```python
from build123d import *

# Parameters (mm, degrees)
F0_W     = 220
F0_H     = 163.86598641
F1_DEPTH = 25.4
F2_W     = 175.2
F2_H     = 30
F3_DEPTH = 57.15


# Not quite as in the source:
# - a feature names something its author has since deleted; it is built from what else it names


with BuildPart() as f1:
    # F0 (on Front) → F1 (new body)
    with BuildSketch(Plane.XZ):
        with Locations((1.3140309602, -1.7520450056)):
            Rectangle(F0_W, F0_H)
    extrude(amount=F1_DEPTH)

    # F2 (on face) → F3 (cut)
    with BuildSketch(Plane.XZ.offset(25.4)):
        with Locations((1.3140309602, 65.1809481994)):
            Rectangle(F2_W, F2_H)
    extrude(amount=-F3_DEPTH, mode=Mode.SUBTRACT)


solid = f1.part
```
Work out the finished part from the listing and answer in its coordinate system (mm). A direction names the side the tool comes from. Give positions to 0.01 mm unless a question says otherwise; leave off trailing zeros. Order: outer loops, then holes, each group sorted by start corner. A loop starts at its lowest first (then second) coordinate and runs counter-clockwise, first axis right, second up. Notation, with made-up numbers: M 80,3 L 106,3 A8 ccw 106,16 Z; hole C 53,-17.75 d10. An arc over 180 degrees is marked long. Return JSON: item names as keys, results as strings.
1) Straight lines are drawn through the part: line 1 along X through (y, z) = (-8, 60); line 2 along Z through (x, y) = (-35, -4.5). For each, find the intervals that lie inside material, in ascending order. Write a range as [from, to].
Resolved:
{"line 1": "[-108.69, -86.29], [88.91, 111.31]", "line 2": "[-83.69, 50.18]"}
2) Section A-A, the plane y = -22.5 is taken. Write down the section's boundary in (x, z), plus the area to 3 significant figures.
Resolved:
{"outline": "M -108.69,-83.69 L 111.31,-83.69 L 111.31,80.18 L 88.91,80.18 L 88.91,50.18 L -86.29,50.18 L -86.29,80.18 L -108.69,80.18 Z", "area": "30,800 mm^2"}
3) A tool of negligible diameter and unlimited length cuts with its end or side. For faces 5 (the flat face through (-86.286, -13, 65)), 6 (the flat face through (111.314, -13, -3)), from which of +Z, -Z, +X, -X, +Y, -Y can it reach the whole face along a straight path? Write none if from no direction.
Resolved:
{"face 5": "+Z, +Y, -Y", "face 6": "+Z, -Z, +X, +Y, -Y"}
4) This flat-tipped pin is pushed along its axis until it touches: pin 1 (5 mm diameter, centred on x = -69, y = -21, fed in from +Z). Where does it stop, or does it pass through?
Resolved:
{"pin 1": "z = 50.18"}
5) For a pull along X with two mould halves and no side action, classify faces 1 (the flat face through (-108.686, -13, -3)), 2 (the flat face through (100, -13, 80.181)), 3 (the flat face through (88.914, -13, 65)), 4 (the flat face through (0, -13, 50.181)) as +X half, -X half, draft (parallel to the pull), parting line (faces both ways), or undercut.
Resolved:
{"face 1": "-X half", "face 2": "draft", "face 3": "undercut", "face 4": "undercut"}
6) Section B-B, the plane x = -49.5 is taken. Write down the section's boundary in (y, z), plus the area to 3 significant figures.
Resolved:
{"outline": "M -25.4,-83.69 L 0,-83.69 L 0,50.18 L -25.4,50.18 Z", "area": "3,400 mm^2"}
